Geometry: see drawing. Coordinates: mm, zero at the bounding-box minimum. Round coordinates to 2 decimals unless told otherwise and drop trailing zeros. Write each loop counter-clockwise with the first axis right and the second up, starting at its lowest first coordinate (ties: lowest second). Pieces come first, ordered by that corner, then holes. Notation, with made-up numbers: (59.25, 55.25) -> (66.25, 55.25) arc R24 cw to (66.25, 78.25) -> close; hole circle Ø6 at (45, 20.5). An arc over 180 degrees is marked (long way). Use CSV: the item, a comma, the result in double quotes.
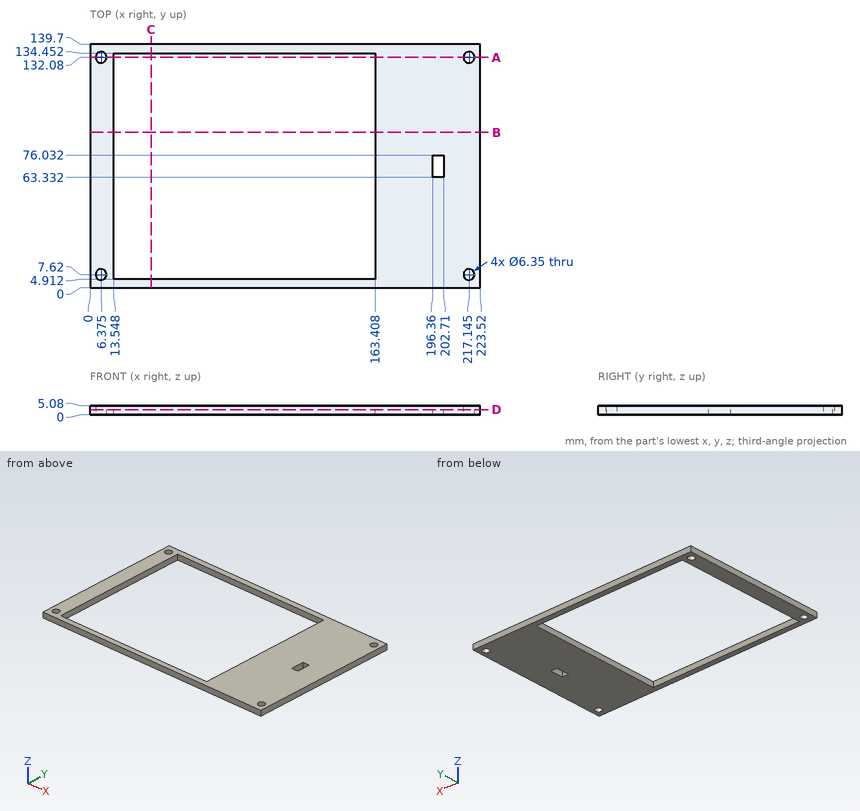
Item 1: Section query C-C on x = 35. Return the cut outline in (y, z), plus the area to 3 significant figures.
Worked answers:
outline,"(0, 0) -> (4.91, 0) -> (4.91, 5.08) -> (0, 5.08) -> close; (134.45, 0) -> (139.7, 0) -> (139.7, 5.08) -> (134.45, 5.08) -> close"
area,"51.6 mm²"
Item 2: Section query B-B on y = 89. Return the cut outline in (x, z).
Worked answers:
outline,"(0, 0) -> (13.55, 0) -> (13.55, 5.08) -> (0, 5.08) -> close; (163.41, 0) -> (223.52, 0) -> (223.52, 5.08) -> (163.41, 5.08) -> close"
Item 3: Section query A-A on y = 132.08. Return the cut outline in (x, z), plus the area to 3 significant figures.
Worked answers:
outline,"(0, 0) -> (3.2, 0) -> (3.2, 5.08) -> (0, 5.08) -> close; (9.55, 0) -> (13.55, 0) -> (13.55, 5.08) -> (9.55, 5.08) -> close; (163.41, 0) -> (213.97, 0) -> (213.97, 5.08) -> (163.41, 5.08) -> close; (220.32, 0) -> (223.52, 0) -> (223.52, 5.08) -> (220.32, 5.08) -> close"
area,"310 mm²"
Item 4: Line query: line 1 (X direction, y = 132.08, z = 3.75); line 2 (Y direction, x = 31, z = 3); line 3 (X direction, y = 68, z = 2.35). Output: solid intervals per line, ascending.
Worked answers:
line 1,"x = 0 to 3.2, 9.55 to 13.55, 163.41 to 213.97, 220.32 to 223.52"
line 2,"y = 0 to 4.91, 134.45 to 139.7"
line 3,"x = 0 to 13.55, 163.41 to 196.36, 202.71 to 223.52"
Item 5: Section query D-D on z = 2.85. Give the number of separate pieces and of enclosed holes in the cut face, plus the area to 3 significant figures.
Worked answers:
separate pieces,"1"
enclosed holes,"6"
area,"11,600 mm²"
